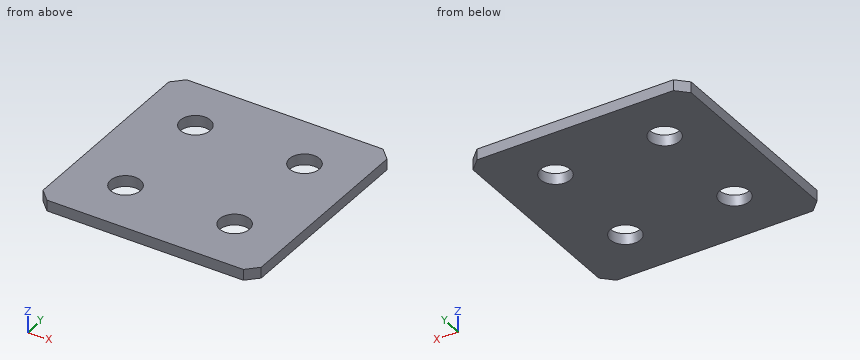
from build123d import *

# Parameters (mm, degrees)
SKETCH_1_W        = 40
SKETCH_1_H        = 40
EXTRUDE_1_DEPTH   = 2
CHAMFER_1_SIZE    = 2
HOLE_WIZARD_M51_D = 5.5


with BuildPart() as part:
    # Эскиз1 → Бобышка-Вытянуть1 (new body)
    with BuildSketch(Plane.XY):
        Rectangle(SKETCH_1_W, SKETCH_1_H)
    extrude(amount=EXTRUDE_1_DEPTH)

    # Фаска1
    chamfer_1_edges = [part.edges().sort_by_distance(p)[0] for p in [
        (20, -20, 1),
        (-20, -20, 1),
        (-20, 20, 1),
        (20, 20, 1),
    ]]
    chamfer(chamfer_1_edges, length=CHAMFER_1_SIZE)

    # Отверстие с зазором M51 (through all)
    with Locations(Plane.XY.offset(2)):
        with Locations((-10, 10), (10, 10), (-10, -10), (10, -10), (-10, 30), (10, 30), (10, -30), (-10, -30)):
            Hole(HOLE_WIZARD_M51_D / 2)


solid = part.part
Design review of the part built by this model. Coordinates are the model's own, in mm. Coordinates: 2 decimals unless noted, no trailing zeros. Write each loop counter-clockwise with the first axis right and the second up, starting at its lowest first coordinate (ties: lowest second). Pieces come first, ordered by that corner, then holes. Notation, with made-up numbers: (-37, -24.75) -> (6, -24.75) arc R23 cw to (6, 1.25) -> close; hole circle Ø10 at (34.25, 1). An arc over 180 degrees is marked (long way). Write each question's results on one line, items separated by ' | '. Start each with the question number.
(1) Take a section at B-B on y = -10. Write out the cut boundary in (x, z), and give its area (3 significant figures).
(2) Clearance check with a flat-ended pin moving along its axis: P1, Ø4.5, axis at x = -10, y = 10, coming from the +Z side. State where the tip first meets the part, or that it passes through.
(3) For line 1 along Y through (x, z) = (10, 1.05); line 2 along X through (y, z) = (10.5, 1.35); line 3 along Y through (x, z) = (-11, 1), list the stretches that pass through material, from the lowest coordinate up. Write a range as from..to.
(4) Take a section at A-A on z = 0.75. Write out the cut boundary in (x, y), and give its area (3 significant figures).
Results found:
1) outline: (-20, 0) -> (-12.75, 0) -> (-12.75, 2) -> (-20, 2) -> close; (-7.25, 0) -> (7.25, 0) -> (7.25, 2) -> (-7.25, 2) -> close; (12.75, 0) -> (20, 0) -> (20, 2) -> (12.75, 2) -> close | area: 58.0 mm2
2) P1: passes through
3) line 1: y = -20..-12.75, -7.25..7.25, 12.75..20 | line 2: x = -20..-12.7, -7.3..7.3, 12.7..20 | line 3: y = -20..-12.56, -7.44..7.44, 12.56..20
4) outline: (-20, -18) -> (-18, -20) -> (18, -20) -> (20, -18) -> (20, 18) -> (18, 20) -> (-18, 20) -> (-20, 18) -> close; hole circle Ø5.5 at (-10, -10); hole circle Ø5.5 at (-10, 10); hole circle Ø5.5 at (10, -10); hole circle Ø5.5 at (10, 10) | area: 1,500 mm2
